Work out the finished part from the listing and answer in its coordinate system (mm). Give positions to 0.01 mm unless a question says otherwise; leave off trailing zeros. Order: outer loops, then holes, each group sorted by start corner. A loop starts at its lowest first (then second) coordinate and runs counter-clockwise, first axis right, second up.
```python
from build123d import *

# Parameters (mm, degrees)
SZKIC1_W                    = 66.4
SZKIC1_H                    = 56.4
SZKIC1_R                    = 19.05
SZKIC1_R_2                  = 2.5
DODANIE_WYCI_GNI_CIE1_DEPTH = 5
OTW_R_GWINTOWANY_M41_D      = 3.3
OTW_R_GWINTOWANY_M42_D      = 3.3


with BuildPart() as part:
    # Szkic1 → Dodanie-wyciągnięcie1 (new body)
    with BuildSketch(Plane(origin=(0, 0, 0), x_dir=(1, 0, 0), z_dir=(0, 1, 0))):
        with Locations((33.2, 28.2)):
            Rectangle(SZKIC1_W, SZKIC1_H)
        with Locations(Location((33.2, 28.2, 0), (0, 0, 270))):
            Circle(SZKIC1_R, mode=Mode.SUBTRACT)
        with Locations(Location((9.63, 51.77, 0), (0, 0, 270))):
            Circle(SZKIC1_R_2, mode=Mode.SUBTRACT)
        with Locations(Location((56.77, 51.77, 0), (0, 0, 90))):
            Circle(SZKIC1_R_2, mode=Mode.SUBTRACT)
        with Locations(Location((56.77, 4.63, 0), (0, 0, 270))):
            Circle(SZKIC1_R_2, mode=Mode.SUBTRACT)
        with Locations(Location((9.63, 4.63, 0), (0, 0, 90))):
            Circle(SZKIC1_R_2, mode=Mode.SUBTRACT)
    extrude(amount=DODANIE_WYCI_GNI_CIE1_DEPTH)

    # Otwór gwintowany M41 (through all)
    with Locations(Plane(origin=(2.5, 5, -51.77), x_dir=(0, 0, 1), z_dir=(0, 1, 0))):
        with Locations((0, 0)):
            Hole(OTW_R_GWINTOWANY_M41_D / 2)

    # Otwór gwintowany M42 (through all)
    with Locations(Plane(origin=(63.9, 5, -51.77), x_dir=(0, 0, 1), z_dir=(0, 1, 0))):
        with Locations((0, 0), (47.14, 0), (47.14, -61.4)):
            Hole(OTW_R_GWINTOWANY_M42_D / 2)


solid = part.part
```
1. Straight lines are drawn through the part: probe 1 along X at (y, z) = (2.8, -51.77); probe 2 along Z at (x, y) = (64, 0.8); probe 3 along Z at (x, y) = (33.5, 1.5). For each, find the intervals that lie inside material, in ascending order.
Findings below:
probe 1: x = 0 to 0.85, 4.15 to 7.13, 12.13 to 54.27, 59.27 to 62.25, 65.55 to 66.4
probe 2: z = -56.4 to -53.42, -50.12 to -6.28, -2.98 to 0
probe 3: z = -56.4 to -47.25, -9.15 to 0
2. The part is cut by section B-B (x = 9.63). Write down the section's boundary in (y, z), then the cut area to 3 significant figures.
Findings below:
outline: (0, -56.4) - (5, -56.4) - (5, -54.27) - (0, -54.27) - close; (0, -49.27) - (5, -49.27) - (5, -7.13) - (0, -7.13) - close; (0, -2.13) - (5, -2.13) - (5, 0) - (0, 0) - close
area: 232 mm2
3. The part is cut by section D-D (y = 1.55). State how many separate pieces and enclosed holes the cut face has, then the cut area to 3 significant figures.
Findings below:
separate pieces: 1
enclosed holes: 9
area: 2,490 mm2
4. Given P1, Ø2.5, axis at x = 63.9, z = -51.77, coming from the -Y side, flat-ended and moving along its own axis, determine where the tip first touches the part or whether it passes through.
Findings below:
P1: passes through
5. The mould has two halves that part along Z. Classify faces 1 (the face through (33, 2, -56.4)), 2 (the face through (11.85, 2.46, -5.78)), 3 (the face through (32.7, 5, -47.4)): pulls with the +Z half, pulls with the -Z half, needs draft (parallel to the pull), parting line crosses it, or undercut.
Findings below:
face 1: pulls with the -Z half
face 2: undercut
face 3: needs draft
6. The part is cut by section A-A (z = -4.63). Write down the section's boundary in (x, y), then the cut area to 3 significant figures.
Findings below:
outline: (0, 0) - (0.85, 0) - (0.85, 5) - (0, 5) - close; (4.15, 0) - (7.13, 0) - (7.13, 5) - (4.15, 5) - close; (12.13, 0) - (54.27, 0) - (54.27, 5) - (12.13, 5) - close; (59.27, 0) - (62.25, 0) - (62.25, 5) - (59.27, 5) - close; (65.55, 0) - (66.4, 0) - (66.4, 5) - (65.55, 5) - close
area: 249 mm2
7. The part is cut by section C-C (z = -28.2). Write down the section's boundary in (x, y).
Findings below:
outline: (0, 0) - (14.15, 0) - (14.15, 5) - (0, 5) - close; (52.25, 0) - (66.4, 0) - (66.4, 5) - (52.25, 5) - close
